Read the model definition and answer for the solid it produces. Units are mm, in the model's axes. A direction names the side the tool comes from. Coordinates: 2 decimals unless noted, no trailing zeros. Write each loop counter-clockwise with the first axis right and the second up, starting at its lowest first coordinate (ties: lowest second). Pieces come first, ordered by that corner, then holes.
Item 1: Section D-D (z = 14) is taken. Give the vertices of the cut face in (x, y), then the cut area to 3 significant figures.
Item 2: Straight lines are drawn through the part: probe 1 along X at (y, z) = (4, 32); probe 2 along Z at (x, y) = (47.5, 3.75); probe 3 along Z at (x, y) = (3, 2.6). For each, find the intervals that lie inside material, in ascending order.
Item 3: Section C-C (y = 3.2) is taken. State how many separate pieces and enclosed holes the cut face has, then the cut area to 3 significant figures.
Item 4: A tool of negligible diameter and unlimited length cuts with its end or side. For faces 4 (the face through (0, 3, 22.679)), 5 (the face through (-1, 5, 31)), from which of +Z, -Z, +X, -X, +Y, -Y can it reach the whole face along a straight path? Write none if from no direction.
Item 5: Determine the mould class of faces 1 (the face through (-29.93, 2.54, 14.14)), 2 (the face through (-53.5, 3, 72)), 3 (the face through (-19.93, 2.54, 13.9)) for opening direction Z: released by +Z, released by -Z, zero draft, split by the parting line, or undercut.
Item 6: This flat-tipped pin is pushed along its axis until it touches: P1, Ø1, axis at x = -55.5, z = 65.5, coming from the -Y side. Where does it stop, or does it pass through?
Item 7: Section A-A (z = 72.5) is taken. Give the vertices of the cut face in (x, y), then the cut area to 3 significant figures.
Item 8: Section B-B (x = -62) is taken. Give the vertices of the cut face in (y, z), then the cut area to 3 significant figures.
from build123d import *

# Parameters (mm, degrees)
SKETCH1_W               = 139
SKETCH1_H               = 160
BOSS_EXTRUDE1_DEPTH     = 5
SKETCH2_W               = 16
SKETCH2_H               = 16
CUT_EXTRUDE1_DEPTH      = 107.090763029
SKETCH3_R               = 2.2
CUT_EXTRUDE2_DEPTH      = 107.090763029
SKETCH4_R               = 2.2
CUT_EXTRUDE3_DEPTH      = 107.090763029
LPATTERN1_COUNT         = 4
LPATTERN1_PITCH         = 35
MIRROR2_COPY_1_SKETCH_R = 2.2
MIRROR2_COPY_1_DEPTH    = 107.090763029
MIRROR2_COPY_2_SKETCH_R = 2.2
MIRROR2_COPY_2_DEPTH    = 107.090763029
MIRROR2_COPY_3_SKETCH_R = 2.2
MIRROR2_COPY_3_DEPTH    = 107.090763029
SKETCH5_R               = 2.2
CUT_EXTRUDE4_DEPTH      = 107.090763029
CUT_EXTRUDE5_DEPTH      = 107.090763029
SKETCH9_W               = 139
SKETCH9_H               = 80
CUT_EXTRUDE6_DEPTH      = 10


with BuildPart() as part:
    # Sketch1 → Boss-Extrude1 (new body)
    with BuildSketch(Plane(origin=(0, 0, 0), x_dir=(1, 0, 0), z_dir=(0, 1, 0))):
        Rectangle(SKETCH1_W, SKETCH1_H)
    extrude(amount=BOSS_EXTRUDE1_DEPTH)

    # Sketch2 → Cut-Extrude1 (cut, through all)
    with BuildSketch(Plane(origin=(0, 5, 0), x_dir=(1, 0, 0), z_dir=(0, 1, 0))):
        with Locations((-61.5, -72)):
            Rectangle(SKETCH2_W, SKETCH2_H)
    cut_extrude1 = extrude(amount=-CUT_EXTRUDE1_DEPTH, mode=Mode.SUBTRACT)

    # Mirror1: Cut-Extrude1 across plane
    add(cut_extrude1.mirror(Plane(origin=(0, 0, 0), x_dir=(0, 0, 1), z_dir=(1, 0, 0))), mode=Mode.SUBTRACT)

    # Sketch3 → Cut-Extrude2 (cut, through all)
    with BuildSketch(Plane(origin=(0, 5, 0), x_dir=(1, 0, 0), z_dir=(0, 1, 0))):
        with Locations(Location((0, -72.5, 0), (0, 0, 270))):
            Circle(SKETCH3_R)
        with Locations(Location((-25, -72.5, 0), (0, 0, 270))):
            Circle(SKETCH3_R)
        with Locations(Location((25, -72.5, 0), (0, 0, 270))):
            Circle(SKETCH3_R)
    extrude(amount=-CUT_EXTRUDE2_DEPTH, mode=Mode.SUBTRACT)

    # Sketch4 → Cut-Extrude3 (cut, through all)
    with BuildSketch(Plane(origin=(0, 5, 0), x_dir=(1, 0, 0), z_dir=(0, 1, 0))):
        with Locations(Location((-62, -49, 0), (0, 0, 270))):
            Circle(SKETCH4_R)
    cut_extrude3 = extrude(amount=-CUT_EXTRUDE3_DEPTH, mode=Mode.SUBTRACT)

    # LPattern1: Cut-Extrude3 ×4
    with Locations(*[(0, 0, -i * LPATTERN1_PITCH) for i in range(1, LPATTERN1_COUNT)]):
        add(cut_extrude3, mode=Mode.SUBTRACT)

    # Mirror2: Cut-Extrude3 across plane
    add(cut_extrude3.mirror(Plane(origin=(0, 0, 0), x_dir=(0, 0, 1), z_dir=(1, 0, 0))), mode=Mode.SUBTRACT)

    # Mirror2 copy 1 sketch → Mirror2 copy 1 (cut, through all)
    with BuildSketch(Plane(origin=(0, 5, -35), x_dir=(-1, 0, 0), z_dir=(0, 1, 0))):
        with Locations((-62, 49)):
            Circle(MIRROR2_COPY_1_SKETCH_R)
    extrude(amount=-MIRROR2_COPY_1_DEPTH, mode=Mode.SUBTRACT)

    # Mirror2 copy 2 sketch → Mirror2 copy 2 (cut, through all)
    with BuildSketch(Plane(origin=(0, 5, -70), x_dir=(-1, 0, 0), z_dir=(0, 1, 0))):
        with Locations((-62, 49)):
            Circle(MIRROR2_COPY_2_SKETCH_R)
    extrude(amount=-MIRROR2_COPY_2_DEPTH, mode=Mode.SUBTRACT)

    # Mirror2 copy 3 sketch → Mirror2 copy 3 (cut, through all)
    with BuildSketch(Plane(origin=(0, 5, -105), x_dir=(-1, 0, 0), z_dir=(0, 1, 0))):
        with Locations((-62, 49)):
            Circle(MIRROR2_COPY_3_SKETCH_R)
    extrude(amount=-MIRROR2_COPY_3_DEPTH, mode=Mode.SUBTRACT)

    # Sketch5 → Cut-Extrude4 (cut, through all)
    with BuildSketch(Plane(origin=(0, 5, 0), x_dir=(1, 0, 0), z_dir=(0, 1, 0))):
        with Locations(Location((-47.5, -32, 0), (0, 0, 270))):
            Circle(SKETCH5_R)
        with Locations(Location((-47.5, -7, 0), (0, 0, 270))):
            Circle(SKETCH5_R)
    cut_extrude4 = extrude(amount=-CUT_EXTRUDE4_DEPTH, mode=Mode.SUBTRACT)

    # Mirror3: Cut-Extrude4 across plane
    add(cut_extrude4.mirror(Plane(origin=(0, 0, 0), x_dir=(0, 0, 1), z_dir=(1, 0, 0))), mode=Mode.SUBTRACT)

    # Sketch6 → Cut-Extrude5 (cut, through all)
    with BuildSketch(Plane(origin=(0, 5, 0), x_dir=(1, 0, 0), z_dir=(0, 1, 0))):
        Polygon((0, 50), (-10, 32.679491924), (10, 32.679491924), align=None)
        Polygon((15, 50), (25, 32.679491924), (35, 50), align=None)
        Polygon((-25, 32.679491924), (-35, 50), (-15, 50), align=None)
        Polygon((25, 22.679491924), (35, 5.358983849), (15, 5.358983849), align=None)
        Polygon((-10, 22.679491924), (10, 22.679491924), (0, 5.358983849), align=None)
        Polygon((-15, 5.358983849), (-25, 22.679491924), (-35, 5.358983849), align=None)
        Polygon((15, -5.358983849), (25, -22.679491924), (35, -5.358983849), align=None)
        Polygon((0, -5.358983849), (-10, -22.679491924), (10, -22.679491924), align=None)
        Polygon((-35, -5.358983849), (-15, -5.358983849), (-25, -22.679491924), align=None)
        Polygon((25, -32.679491924), (35, -50), (15, -50), align=None)
        Polygon((-10, -32.679491924), (10, -32.679491924), (0, -50), align=None)
        Polygon((-15, -50), (-25, -32.679491924), (-35, -50), align=None)
    extrude(amount=-CUT_EXTRUDE5_DEPTH, mode=Mode.SUBTRACT)

    # Sketch9 → Cut-Extrude6 (cut)
    with BuildSketch(Plane(origin=(0, 5, 0), x_dir=(1, 0, 0), z_dir=(0, 1, 0))):
        with Locations((0, 40)):
            Rectangle(SKETCH9_W, SKETCH9_H)
    extrude(amount=-CUT_EXTRUDE6_DEPTH, mode=Mode.SUBTRACT)


solid = part.part
Established:
1. outline: (-69.5, 0) - (-64.2, 0) - (-64.2, 5) - (-69.5, 5) - close; (-59.8, 0) - (-30.01, 0) - (-30.01, 5) - (-59.8, 5) - close; (-19.99, 0) - (-4.99, 0) - (-4.99, 5) - (-19.99, 5) - close; (4.99, 0) - (19.99, 0) - (19.99, 5) - (4.99, 5) - close; (30.01, 0) - (59.8, 0) - (59.8, 5) - (30.01, 5) - close; (64.2, 0) - (69.5, 0) - (69.5, 5) - (64.2, 5) - close
1. area: 501 mm2
2. probe 1: x = -69.5 to -49.7, -45.3 to 45.3, 49.7 to 69.5
2. probe 2: z = 0 to 4.8, 9.2 to 29.8, 34.2 to 80
2. probe 3: z = 0 to 10.56, 22.68 to 32.68, 44.8 to 80
3. separate pieces: 1
3. enclosed holes: 17
3. area: 9,400 mm2
4. face 4: +Y, -Y
4. face 5: +Z, -Z, +X, -X, +Y
5. face 1: undercut
5. face 2: zero draft
5. face 3: undercut
6. P1: passes through
7. outline: (-53.5, 0) - (-27.2, 0) - (-27.2, 5) - (-53.5, 5) - close; (-22.8, 0) - (-2.2, 0) - (-2.2, 5) - (-22.8, 5) - close; (2.2, 0) - (22.8, 0) - (22.8, 5) - (2.2, 5) - close; (27.2, 0) - (53.5, 0) - (53.5, 5) - (27.2, 5) - close
7. area: 469 mm2
8. outline: (0, 0) - (5, 0) - (5, 11.8) - (0, 11.8) - close; (0, 16.2) - (5, 16.2) - (5, 46.8) - (0, 46.8) - close; (0, 51.2) - (5, 51.2) - (5, 64) - (0, 64) - close
8. area: 276 mm2
